For this review, take the finished solid that the model builds, in its own axes (mm). Give positions to 0.01 mm unless a question says otherwise; leave off trailing zeros. Write each loop counter-clockwise with the first axis right and the second up, starting at its lowest first coordinate (ties: lowest second). Pieces come first, ordered by that corner, then holes. Notation, with made-up numbers: (39, 22.5) -> (56, 22.5) arc R15 cw to (56, 36.5) -> close; hole circle Ø7 at (11.5, -1). An arc over 180 degrees is marked (long way). Return JSON: item names as keys, results as strings.
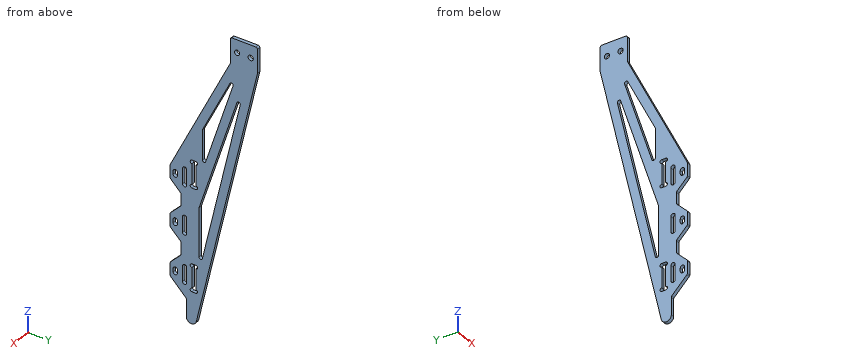
from build123d import *

# Parameters (mm, degrees)
SKETCH_1_R      = 1.55
EXTRUDE_1_DEPTH = 2
FILLET_1_R      = 1
FILLET_2_R      = 3


with BuildPart() as part:
    # 草图1 → 凸台-拉伸1 (new body)
    with BuildSketch(Plane(origin=(0, 0, 0), x_dir=(0, 0, -1), z_dir=(1, 0, 0))):
        Polygon((7.5, 12), (-7.5, 12), (-7.5, -4), (7.5, -4), (79.182692308, -39.5), (87.182692308, -39.5), (93.682692308, -33), (100.682692308, -33), (107.182692308, -39.5), (115.182692308, -39.5), (121.682692308, -33), (129.1, -33), (135.6, -39.5), (143.6, -39.5), (153.1, -30), (190.043283582, -30), align=None)
        with BuildLine():
            Line((78.682692308, -29.75), (87.682692308, -29.75))
            ThreePointArc((87.682692308, -29.75), (88.932692308, -31), (87.682692308, -32.25))
            Line((87.682692308, -32.25), (78.682692308, -32.25))
            ThreePointArc((78.682692308, -32.25), (77.432692308, -31), (78.682692308, -29.75))
        make_face(mode=Mode.SUBTRACT)
        with BuildLine():
            Line((106.682692308, -29.75), (115.682692308, -29.75))
            ThreePointArc((115.682692308, -29.75), (116.932692308, -31), (115.682692308, -32.25))
            Line((115.682692308, -32.25), (106.682692308, -32.25))
            ThreePointArc((106.682692308, -32.25), (105.432692308, -31), (106.682692308, -29.75))
        make_face(mode=Mode.SUBTRACT)
        with BuildLine():
            Line((135.1, -29.75), (144.1, -29.75))
            ThreePointArc((144.1, -29.75), (145.35, -31), (144.1, -32.25))
            Line((144.1, -32.25), (135.1, -32.25))
            ThreePointArc((135.1, -32.25), (133.85, -31), (135.1, -29.75))
        make_face(mode=Mode.SUBTRACT)
        with BuildLine():
            Line((86, -26.65), (74, -26.65))
            ThreePointArc((74, -26.65), (72.95, -27.7), (71.9, -26.65))
            Line((71.9, -26.65), (71.9, -24.35))
            ThreePointArc((71.9, -24.35), (72.95, -23.3), (74, -24.35))
            Line((74, -24.35), (86, -24.35))
            ThreePointArc((86, -24.35), (87.05, -23.3), (88.1, -24.35))
            Line((88.1, -24.35), (88.1, -26.65))
            ThreePointArc((88.1, -26.65), (87.05, -27.7), (86, -26.65))
        make_face(mode=Mode.SUBTRACT)
        with BuildLine():
            Line((146, -26.65), (134, -26.65))
            ThreePointArc((134, -26.65), (132.95, -27.7), (131.9, -26.65))
            Line((131.9, -26.65), (131.9, -24.35))
            ThreePointArc((131.9, -24.35), (132.95, -23.3), (134, -24.35))
            Line((134, -24.35), (146, -24.35))
            ThreePointArc((146, -24.35), (147.05, -23.3), (148.1, -24.35))
            Line((148.1, -24.35), (148.1, -26.65))
            ThreePointArc((148.1, -26.65), (147.05, -27.7), (146, -26.65))
        make_face(mode=Mode.SUBTRACT)
        Polygon((52.083732258, -20.5), (7, 1.827181689), (75.890858402, -20.5), align=None, mode=Mode.SUBTRACT)
        Polygon((97.974573659, -22.5), (7, 6.984403045), (135.147136815, -22.5), align=None, mode=Mode.SUBTRACT)
        Circle(SKETCH_1_R, mode=Mode.SUBTRACT)
        with Locations((0, 8)):
            Circle(SKETCH_1_R, mode=Mode.SUBTRACT)
        with BuildLine():
            Line((138.6, -35.25), (140.6, -35.25))
            ThreePointArc((140.6, -35.25), (141.85, -36.5), (140.6, -37.75))
            Line((140.6, -37.75), (138.6, -37.75))
            ThreePointArc((138.6, -37.75), (137.35, -36.5), (138.6, -35.25))
        make_face(mode=Mode.SUBTRACT)
        with BuildLine():
            ThreePointArc((82.182692308, -37.75), (80.932692308, -36.5), (82.182692308, -35.25))
            Line((82.182692308, -35.25), (84.182692308, -35.25))
            ThreePointArc((84.182692308, -35.25), (85.432692308, -36.5), (84.182692308, -37.75))
            Line((84.182692308, -37.75), (82.182692308, -37.75))
        make_face(mode=Mode.SUBTRACT)
        with BuildLine():
            ThreePointArc((110.182692308, -37.75), (108.932692308, -36.5), (110.182692308, -35.25))
            Line((110.182692308, -35.25), (112.182692308, -35.25))
            ThreePointArc((112.182692308, -35.25), (113.432692308, -36.5), (112.182692308, -37.75))
            Line((112.182692308, -37.75), (110.182692308, -37.75))
        make_face(mode=Mode.SUBTRACT)
    extrude(amount=EXTRUDE_1_DEPTH)

    # 圆角1
    fillet_1_edges = [part.edges().sort_by_distance(p)[0] for p in [
        (1, -33, -121.682692308),
        (1, -39.5, -115.182692308),
        (1, -39.5, -107.182692308),
        (1, -33, -100.682692308),
        (1, -33, -93.682692308),
        (1, -39.5, -87.182692308),
        (1, -39.5, -79.182692308),
        (1, -4, -7.5),
        (1, -4, 7.5),
        (1, 12, 7.5),
        (1, 12, -7.5),
        (1, -30, -153.1),
        (1, -39.5, -143.6),
        (1, -39.5, -135.6),
        (1, -33, -129.1),
        (1, 6.984403045, -7),
        (1, -22.5, -97.974573659),
        (1, -22.5, -135.147136815),
        (1, 1.827181689, -7),
        (1, -20.5, -52.083732258),
        (1, -20.5, -75.890858402),
    ]]
    fillet(fillet_1_edges, radius=FILLET_1_R)

    # 圆角2
    fillet_2_edges = [part.edges().sort_by_distance(p)[0] for p in [
        (1, -30, -190.043283582),
    ]]
    fillet(fillet_2_edges, radius=FILLET_2_R)


solid = part.part
1. Add section A-A, the plane z = -33.5. State the section outline as (x, y) points.
Results found:
{"outline": "(0, -16.88) -> (2, -16.88) -> (2, -11.3) -> (0, -11.3) -> close; (0, -6.76) -> (2, -6.76) -> (2, -1.6) -> (0, -1.6) -> close; (0, 0.89) -> (2, 0.89) -> (2, 6.02) -> (0, 6.02) -> close"}
2. To check wall thickness, follow probe 1 along Y at (x, z) = (1.4, 0); probe 2 along Y at (x, z) = (1.9, -135); probe 3 along Z at (x, y) = (1.8, -34). State the ranges of each line that lie inside material, in increasing order.
Results found:
{"probe 1": "y = -4 to -1.55, 1.55 to 6.45, 9.55 to 12", "probe 2": "y = -38.9 to -32.25, -29.75 to -26.65, -24.35 to -17.34", "probe 3": "z = -149.1 to -130.1, -120.68 to -101.68, -92.68 to -68.08"}
3. Add section B-B, the plane x = 1. Count the separate pieces of the cut face and the enclosed holes in it, plus the area to 3 significant figures.
Results found:
{"separate pieces": "1", "enclosed holes": "12", "area": "2,910 mm²"}
4. For pin 1 (1 mm diameter, centred on x = 1, z = -142.5, fed in from +Y); pin 2 (1 mm diameter, centred on x = 0.5, z = -129, fed in from -Y); pin 3 (1 mm diameter, centred on x = 1, z = -138, fed in from +Y), all flat-tipped, find the tip position at first contact; note any pin that passes through.
Results found:
{"pin 1": "stops at y = -18.95", "pin 2": "stops at y = -33.4", "pin 3": "stops at y = -17.91"}
